Work out the finished part from the listing and answer in its coordinate system (mm). A direction names the side the tool comes from. Give positions to 0.01 mm unless a question says otherwise; leave off trailing zeros. Use a Markdown table: item, result. Add a question column.
Q1. Consider line 1 (Z direction, x = 12.5, y = -104); line 2 (Z direction, x = 2, y = 85); line 3 (X direction, y = 68, z = -6). Determine where each line is inside the solid, lowest interval first.
Q2. Each of these flat-tipped pins is pushed along its axis until it touches: pin 1 Ø5 at (y, z) = (-32.5, -0.5) entering from +X; pin 2 Ø5 at (y, z) = (37.5, 0.5) entering from -X. Where does it stop, or does it pass through?
Q3. For a pull along Z with two mould halves and no side action, classify faces 1 (the face through (0, 125, 0)), 2 (the face through (7, -2, 1)), 3 (the face through (0, -2, 7.5)) as pulls with the +Z half, pulls with the -Z half, needs draft (parallel to the pull), parting line crosses it, or undercut.
Q4. For faces 4 (the face through (-7, -2, 1)), 5 (the face through (0, -2, -1.5)), 6 (the face through (9, -2, 0)), 7 (the face through (-9, -2, 0)), 8 (the face through (-9, -2, -7.5)), determine the directions among +Z, -Z, +X, -X, +Y, -Y from which every point of the face is accessible in a straight line to the end or side of a thin tool.
Autodesk Inventor part; units mm, degrees
ref_plane "YZ Plane" through (0, 0, 0) normal (1, 0, 0) x (0, 1, 0)
ref_plane "XZ Plane" through (0, 0, 0) normal (0, 1, 0) x (-1, 0, 0)
ref_plane "XY Plane" through (0, 0, 0) normal (0, 0, 1) x (1, 0, 0)
sketch "Esboço1" plane through (0, 0, 0) normal (0, 1, 0) x (-1, 0, 0)
  line L0 (-15, 7.5) -> (15, 7.5) construction
  line L1 (15, 7.5) -> (15, -7.5) construction
  line L2 (15, -7.5) -> (-15, -7.5) construction
  line L3 (-15, -7.5) -> (-15, 7.5) construction
  line L4 (15, 7.5) -> (-15, -7.5) construction
  line L5 (0, 7.5) -> (14, 7.5)
  arc A0 (15, 6.5) -> (14, 7.5) centre (14, 6.5) ccw
  line L6 (15, 6.5) -> (15, 3.6)
  line L7 (15, 3.6) -> (14.5, 3.6)
  line L8 (14.5, 3.6) -> (14.5, 3.1)
  line L9 (14.5, 3.1) -> (13, 3.1)
  line L10 (13, 3.1) -> (13, 5.6)
  line L11 (12.1786, 5.983) -> (9.1786, 3.4657)
  arc A1 (13, 5.6) -> (12.1786, 5.983) centre (12.5, 5.6) ccw
  arc A2 (9.1786, 3.4657) -> (9, 3.0827) centre (9.5, 3.0827) ccw
  line L12 (14, -7.5) -> (3.6, -7.5)
  line L13 (15, -3.6) -> (15, -6.5)
  arc A3 (14, -7.5) -> (15, -6.5) centre (14, -6.5) ccw
  line L14 (15, -3.6) -> (14.5, -3.6)
  line L15 (14.5, -3.6) -> (14.5, -3.1)
  line L16 (14.5, -3.1) -> (13, -3.1)
  line L17 (13, -3.1) -> (13, -5.6)
  line L18 (12.1786, -5.983) -> (9.1786, -3.4657)
  arc A4 (12.1786, -5.983) -> (13, -5.6) centre (12.5, -5.6) ccw
  line L19 (9, 3.0827) -> (9, -3.0827)
  arc A5 (9, -3.0827) -> (9.1786, -3.4657) centre (9.5, -3.0827) ccw
  line L20 (0, 5.5) -> (7.1178, 5.5)
  line L21 (0, 5.5) -> (0, 7.5)
  line L22 (13, -3.1) -> (13, 3.1) construction
  line L23 (7, -2.1501) -> (7, 4.0153)
  arc A6 (7.4392, 4.617) -> (7.1178, 5.5) centre (7.1178, 5) ccw
  arc A7 (7.1786, 4.3983) -> (7, 4.0153) centre (7.5, 4.0153) ccw
  line L24 (8.4915, 5.5) -> (7.1178, 5.5) construction
  line L25 (8.4915, 5.5) -> (7.1786, 4.3983) construction
  line L26 (7.1786, 4.3983) -> (7.4392, 4.617)
  line L27 (7, 4.0153) -> (7, -3.6) construction
  line L28 (7, -3.6) -> (3.9407, 0.3082) construction
  arc A8 (6.1063, -2.4583) -> (7, -2.1501) centre (6.5, -2.1501) ccw
  line L29 (6.1063, -2.4583) -> (3.9407, 0.3082)
  line L30 (3.547, 0.5) -> (0, 0.5)
  arc A9 (3.9407, 0.3082) -> (3.547, 0.5) centre (3.547, 0) ccw
  line L31 (0, 0.5) -> (0, -1.5)
  line L32 (0, -1.5) -> (3.0827, -1.5)
  line L33 (3.6, -7.5) -> (3.6, -7)
  line L34 (3.6, -7) -> (3.1, -7)
  line L35 (3.1, -7) -> (3.1, -5.5)
  line L36 (3.1, -5.5) -> (5.6, -5.5)
  line L37 (5.983, -4.6786) -> (3.4657, -1.6786)
  arc A10 (3.4657, -1.6786) -> (3.0827, -1.5) centre (3.0827, -2) ccw
  arc A11 (5.6, -5.5) -> (5.983, -4.6786) centre (5.6, -5) ccw
  line L38 (0, 2.5907) -> (0, -7.5) construction
  point P0 (0, 0)
  point P1 (13, -4.35)
  point P2 (13, 0)
  point P3 (9.0468, 3.294)
  dimension "d14" = 30
  dimension "d15" = 15
  dimension "d22" = 2
  dimension "d23" = 0.5
  dimension "d34" = 2.5
  dimension "d35" = 1
  dimension "d37" = 0.5
  dimension "d38" = 50
  dimension "d41" = 6
  dimension "d45" = 2
  dimension "d46" = 6.2
  dimension "d47" = 2
  dimension "d50" = 0.5
  dimension "d53" = 2
  dimension "d55" = 2
  dimension "d56" = 3.1
  dimension "d59" = 6
  dimension "d60" = 50
  dimension "d62" = 2
  dimension "d64" = 1.4656
extrude "Extrusão1" add sketch "Esboço1" along normal mid plane 250
mirror "Espelhar1" about plane through (0, 0, 0) normal (1, 0, 0) of "Extrusão1"
equation "\"d47\" = d45"
equation "\"Raio_vergadura\" = Espessura"
equation "\"Largura_alívio_de_vergadura\" = Espessura"
equation "\"Profundidade_alívio_de_vergadura\" = 0.5 * Espessura"
equation "\"Tamanho_alívio_de_dobra\" = 4 * Espessura"
equation "\"Remanescente_mínimo\" = 2 * Espessura"
equation "\"Raiodetransição\" = Raio_vergadura"
equation "\"Tamanho_de_raio_de_Jacobi\" = Raio_vergadura"
equation "\"TamanhoFolga\" = Espessura"
Result set:
| question | item | result |
|---|---|---|
| 1 | line 1 | z = -7.5 to -6.1, 6.1 to 7.5 |
| 1 | line 2 | z = -1.5 to 0.5, 5.5 to 7.5 |
| 1 | line 3 | x = -15 to -12.8, -12.2 to -3.1, 3.1 to 12.2, 12.8 to 15 |
| 2 | pin 1 | stops at x = 9 |
| 2 | pin 2 | stops at x = -9 |
| 3 | face 1 | needs draft |
| 3 | face 2 | undercut |
| 3 | face 3 | pulls with the +Z half |
| 4 | face 4 | +Y, -Y |
| 4 | face 5 | -Z, +Y, -Y |
| 4 | face 6 | +X, +Y, -Y |
| 4 | face 7 | -X, +Y, -Y |
| 4 | face 8 | -Z, +X, -X, +Y, -Y |
